Model file for the job. Use its own axes, mm. Coordinates: 2 decimals unless noted, no trailing zeros. Write each loop counter-clockwise with the first axis right and the second up, starting at its lowest first coordinate (ties: lowest second). Pieces come first, ordered by that corner, then holes. Notation, with made-up numbers: M -39,-37.75 L -6,-37.75 A10 ccw -6,-25.75 Z; hole C 26.5,41 d2. An arc over 180 degrees is marked long. One line per question, with ' | ' between items. Start each with the question number.
(1) Wall check: probe 1 along Y at (x, z) = (-87.5, 14.75); probe 2 along Y at (x, z) = (0, 7.75); probe 3 along X at (y, z) = (113, 6.75). Give the ranges that are in metal, low to high.
(2) Two-plate mould, pull along X, no slides. Class faces 1 (the face through (-82.881, 108.085, 11.154)), 2 (the face through (-2, 125, 11)), 3 (the face through (-125, -2, 11)), 4 (the face through (92.119, 108.085, 11.154)): +X half, -X half, draft (parallel to the pull), parting line (faces both ways), or undercut.
(3) Cut at A-A (x = -87.5). Write the cut outline in (y, z), plus the area to 3 significant figures.
(4) Flat gauge pin, fed straight in: pin 1 Ø6 at (x, y) = (0, -85) entering from +Z. Where does the tip first touch, or does it go through?
(5) Cut at C-C (y = -85). Write the cut outline in (x, z), plus the area to 3 significant figures.
(6) Cut at B-B (y = 110). Write the cut outline in (x, z).
from build123d import *

# Parameters (mm, degrees)
ESQUISSE1_W          = 250
ESQUISSE1_H          = 250
BOSS_EXTRU_1_DEPTH   = 22
D_GAGEMENT_M81_D     = 10
D_GAGEMENT_M81_DEPTH = 208
D_GAGEMENT_M81_TIP   = 3.004303095


with BuildPart() as part:
    # Esquisse1 → Boss.-Extru.1 (new body)
    with BuildSketch(Plane.XY):
        Rectangle(ESQUISSE1_W, ESQUISSE1_H)
    extrude(amount=BOSS_EXTRU_1_DEPTH)

    # Dégagement M81
    with Locations(Plane(origin=(0, 110, -30), x_dir=(-1, 0, 0), z_dir=(0, 0, -1))):
        with Locations((-87.5, 0), (87.5, 0), (0, -195)):
            Hole(D_GAGEMENT_M81_D / 2, depth=D_GAGEMENT_M81_DEPTH)
            with Locations((0, 0, -(D_GAGEMENT_M81_DEPTH + D_GAGEMENT_M81_TIP / 2))):  # 118° drill point
                Cone(0, D_GAGEMENT_M81_D / 2, D_GAGEMENT_M81_TIP, mode=Mode.SUBTRACT)


solid = part.part
Filled in:
1) probe 1: -125 to 105, 115 to 125 | probe 2: -125 to -90, -80 to 125 | probe 3: -125 to -91.5, -83.5 to 83.5, 91.5 to 125
2) face 1: undercut | face 2: draft | face 3: -X half | face 4: undercut
3) outline: M -125,0 L 105,0 L 105,22 L -125,22 Z; M 115,0 L 125,0 L 125,22 L 115,22 Z | area: 5,280 mm²
4) pin 1: through
5) outline: M -125,0 L -5,0 L -5,22 L -125,22 Z; M 5,0 L 125,0 L 125,22 L 5,22 Z | area: 5,280 mm²
6) outline: M -125,0 L -92.5,0 L -92.5,22 L -125,22 Z; M -82.5,0 L 82.5,0 L 82.5,22 L -82.5,22 Z; M 92.5,0 L 125,0 L 125,22 L 92.5,22 Z
